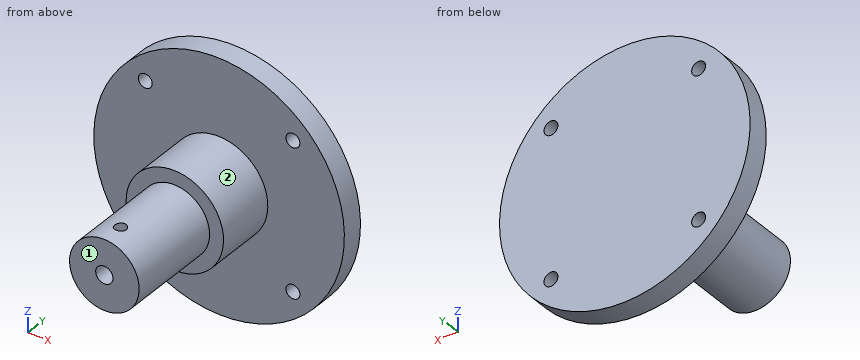
from build123d import *

# Parameters (mm, degrees)
BROCA_DE_ROSQUEAR_PARA_TARRAXA_DE_M62_D = 5
ESBO_O4_R                               = 3.1
CORTE_EXTRUS_O1_DEPTH                   = 18
ESBO_O7_W                               = 2.1
ESBO_O7_H                               = 45
ESBO_O8_R                               = 17.5
ESBO_O8_R_2                             = 12.5
CORTE_EXTRUS_O2_DEPTH                   = 35


with BuildPart() as part:
    # Esboço1 → Revolução1 (revolve)
    with BuildSketch(Plane.XY, mode=Mode.PRIVATE) as revolu_o1_sk:
        Polygon((0, 0), (0, 65), (45, 65), (45, 57), (17.5, 57), (17.5, 0), align=None)
    revolve(revolu_o1_sk.sketch.rotate(Axis((0, 0, 0), (0, 1, 0)), 90), axis=Axis((0, 0, 0), (0, 1, 0)))

    # Broca de rosquear para tarraxa de M62 (through all)
    with Locations(Plane(origin=(0, 65, 0), x_dir=(1, 0, 0), z_dir=(0, 1, 0))):
        with Locations((26.516504294, 26.516504294), (-26.516504294, -26.516504294), (-26.516504294, 26.516504294), (26.516504294, -26.516504294)):
            Hole(BROCA_DE_ROSQUEAR_PARA_TARRAXA_DE_M62_D / 2)

    # Esboço4 → Corte-extrusão1 (cut)
    with BuildSketch(Plane.XZ):
        with Locations(Location((0, 0, 0), (0, 0, 270))):
            Circle(ESBO_O4_R)
    extrude(amount=-CORTE_EXTRUS_O1_DEPTH, mode=Mode.SUBTRACT)

    # Esboço7 → Broca de rosquear para tarraxa de M52 (revolve, cut)
    with BuildSketch(Plane(origin=(0, 8, 0), x_dir=(0, 1, 0), z_dir=(1, 0, 0))):
        with Locations((1.05, 22.5)):
            Rectangle(ESBO_O7_W, ESBO_O7_H)
    revolve(axis=Axis((0, 8, -6.35), (0, 0, 1)), mode=Mode.SUBTRACT)

    # Esboço8 → Corte-extrusão2 (cut)
    with BuildSketch(Plane.XZ):
        with Locations(Location((0, 0, 0), (0, 0, 270))):
            Circle(ESBO_O8_R)
        with Locations(Location((0, 0, 0), (0, 0, 270))):
            Circle(ESBO_O8_R_2, mode=Mode.SUBTRACT)
    extrude(amount=-CORTE_EXTRUS_O2_DEPTH, mode=Mode.SUBTRACT)


solid = part.part
Work out the finished part from the listing and answer in its coordinate system (mm). Face numbers are marked on the shaded views. A direction names the side the tool comes from. Give positions to 0.01 mm unless a question says otherwise; leave off trailing zeros. Order: outer loops, then holes, each group sorted by start corner. A loop starts at its lowest first (then second) coordinate and runs counter-clockwise, first axis right, second up. Notation, with made-up numbers: (32.25, -18) -> (73.25, -18) arc R25 ccw to (73.25, 1) -> close; hole circle Ø11 at (36, 75.5). An arc over 180 degrees is marked (long way). One line per item, written item: value.
Item 1: Find section C-C, the plane x = 27. Give the vertices of the cut face in (y, z).
Answer sheet:
outline: (57, -36) -> (65, -36) -> (65, -28.97) -> (57, -28.97) -> close; (57, -24.06) -> (65, -24.06) -> (65, 24.06) -> (57, 24.06) -> close; (57, 28.97) -> (65, 28.97) -> (65, 36) -> (57, 36) -> close
Item 2: Flat-ended cylindrical pins translate along their axes: P1, Ø4.5, axis at x = -26.52, z = 26.52, coming from the -Y side; P2, Ø5, axis at x = -0.5, y = 38.5, coming from the -Z side; P3, Ø10.5, axis at x = 4.5, z = -1.5, coming from the -Y side; P4, Ø4, axis at x = -12.5, y = 29, coming from the -Z side. Find the tip coordinate at first contact, or state that the pin passes through.
Answer sheet:
P1: through
P2: z = -17.5
P3: y = 0
P4: z = -6.78
Item 3: Find section A-A, the plane x = 0. Give the vertices of the cut face in (y, z), plus the area to 3 significant figures.
Answer sheet:
outline: (0, -12.5) -> (35, -12.5) -> (35, -17.5) -> (57, -17.5) -> (57, -45) -> (65, -45) -> (65, 45) -> (57, 45) -> (57, 17.5) -> (35, 17.5) -> (35, 12.5) -> (10.1, 12.5) -> (10.1, 3.1) -> (18, 3.1) -> (18, -3.1) -> (0, -3.1) -> close; (0, 3.1) -> (5.9, 3.1) -> (5.9, 12.5) -> (0, 12.5) -> close
area: 2,210 mm²
Item 4: Find section B-B, the plane z = 0. Give the vertices of the cut face in (x, y).
Answer sheet:
outline: (-45, 57) -> (-17.5, 57) -> (-17.5, 35) -> (-12.5, 35) -> (-12.5, 0) -> (-3.1, 0) -> (-3.1, 18) -> (3.1, 18) -> (3.1, 0) -> (12.5, 0) -> (12.5, 35) -> (17.5, 35) -> (17.5, 57) -> (45, 57) -> (45, 65) -> (-45, 65) -> close
Item 5: A tool of negligible diameter and unlimited length cuts with its end or side. For the marked faces 1 and 2, from which of +Z, -Z, +X, -X, +Y, -Y can it reach the whole face along a straight path? Write none if from no direction.
Answer sheet:
face 1: +Z, -Z, +X, -X, -Y
face 2: -Y
Item 6: Straight lines are drawn through the part: probe 1 along Z at (x, y) = (0, 5); probe 2 along Y at (x, z) = (0.5, 28); probe 3 along X at (y, z) = (45, -13). For each, find the intervals that lie inside material, in ascending order.
Answer sheet:
probe 1: -12.5 to -3.1, 3.1 to 12.5
probe 2: 57 to 65
probe 3: -11.72 to 11.72
Item 7: Find section D-D, the plane y = 33.5. Give the vertices of the cut face in (x, z).
Answer sheet:
outline: circle Ø25 at (0, 0)
